Read the model definition and answer for the solid it produces. Units are mm, in the model's axes. Coordinates: 2 decimals unless noted, no trailing zeros. Order: outer loops, then holes, each group sorted by start corner. A loop starts at its lowest first (then second) coordinate and runs counter-clockwise, first axis right, second up.
Autodesk Inventor part; units mm, degrees
ref_plane "YZ Plane" through (0, 0, 0) normal (1, 0, 0) x (0, 1, 0)
ref_plane "XZ Plane" through (0, 0, 0) normal (0, 1, 0) x (-1, 0, 0)
ref_plane "XY Plane" through (0, 0, 0) normal (0, 0, 1) x (1, 0, 0)
sketch "Sketch1" plane through (0, 0, 0) normal (0, 1, 0) x (-1, 0, 0)
  line L0 (7.366, 6.1452) -> (7.366, -23.8548)
  line L1 (7.366, -23.8548) -> (0, -23.8548)
  line L2 (6.096, -8.0476) -> (6.096, -9.0212)
  line L3 (0, 0.4868) -> (0, 3.5348)
  line L4 (6.096, 3.5348) -> (6.096, -8.0476)
  line L5 (0, -9.0212) -> (0, -11.8152)
  line L6 (6.096, -12.0692) -> (6.096, -9.0212)
  line L7 (6.096, 3.5348) -> (0, 0.4868)
  line L8 (6.096, -12.0692) -> (0, -9.0212)
  line L9 (0, -23.8548) -> (0, -9.0212)
  line L10 (0, 0.4868) -> (0, 16.3788)
  line L11 (6.096, 13.3308) -> (6.096, 16.3788)
  line L12 (6.096, 13.3308) -> (0, 16.3788)
  line L13 (6.096, 28.9348) -> (6.096, 17.3524)
  line L14 (6.096, 28.9348) -> (0, 25.8868)
  line L15 (6.096, 17.3524) -> (6.096, 16.3788)
  line L16 (6.096, 38.7308) -> (6.096, 41.7788)
  line L17 (6.096, 38.7308) -> (0, 41.7788)
  line L18 (6.096, 54.3348) -> (6.096, 42.7524)
  line L19 (6.096, 54.3348) -> (0, 51.2868)
  line L20 (6.096, 42.7524) -> (6.096, 41.7788)
  line L21 (6.096, 64.1308) -> (6.096, 67.1788)
  line L22 (6.096, 64.1308) -> (0, 67.1788)
  line L23 (6.096, 79.7348) -> (6.096, 68.1524)
  line L24 (6.096, 79.7348) -> (0, 76.6868)
  line L25 (6.096, 68.1524) -> (6.096, 67.1788)
  line L26 (7.366, 6.1452) -> (7.366, 91.622)
  line L27 (7.366, 91.622) -> (0, 91.622)
  line L28 (0, 25.8868) -> (0, 41.7788)
  line L29 (0, 51.2868) -> (0, 67.1788)
  line L30 (0, 76.6868) -> (0, 91.622)
  line L31 (6.096, -4.2672) -> (4.0009, -4.2672) construction
  point P0 (0, 0)
  dimension "d0" = 7.366
  dimension "d8" = 9.508
  dimension "d10" = 3.048
  dimension "d11" = 3.048
  dimension "d12" = 6.096
  dimension "d17" = 25.4
  dimension "d24" = 11.7856
  dimension "d67" = 115.4768
  dimension "d70" = 23.8548
  dimension "d71" = 4.754
extrude "MultipleTeeth" add sketch "Sketch1" along normal blind 19.05
sketch "Sketch2" plane through (0, 0, 0) normal (0, -1, 0) x (1, 0, 0)
  line L0 (0, 0.4868) -> (-6.096, 3.5348) construction
  line L1 (-6.096, 3.5348) -> (-6.096, -12.0692) construction
  line L2 (-6.096, -12.0692) -> (0, -9.0212) construction
  line L3 (0, 16.3788) -> (0, 0.4868)
  line L4 (0, 0.4868) -> (-6.096, 3.5348)
  line L5 (-6.096, -12.0692) -> (0, -9.0212)
  line L6 (-6.096, 3.5348) -> (-6.096, -12.0692)
  line L7 (-6.096, -12.0692) -> (-6.096, 3.5348)
  line L8 (0, -9.0212) -> (-6.096, -12.0692)
  line L9 (-7.366, -23.8548) -> (-7.366, 91.622)
  line L10 (-7.366, -59.508) -> (-7.366, -32.8548)
  line L11 (-7.366, -23.8548) -> (0, -23.8548)
  line L12 (-7.366, 91.622) -> (0, 91.622)
  line L13 (-7.366, -55.8503) -> (-7.366, -40.458) construction
  line L14 (0, -43.0234) -> (0, -59.508) construction
  line L15 (-6.096, -62.0648) -> (0, -62.0648) construction
  line L16 (0, -32.8548) -> (0, -37.6258)
  line L17 (0, -49.9828) -> (0, -62.0648)
  line L18 (0, -62.0648) -> (0, -59.508)
  line L19 (0, -32.8548) -> (-7.366, -32.8548) construction
  line L20 (0, -51.9048) -> (-7.366, -51.9048) construction
  line L21 (0, -42.3798) -> (-7.366, -42.3798) construction
  line L22 (-6.096, -12.0692) -> (-6.096, -62.0648) construction
  line L23 (0, -37.6258) -> (-6.096, -34.5778)
  line L24 (-6.096, -50.1818) -> (-6.096, -34.5778)
  line L25 (0, -47.1338) -> (-6.096, -50.1818)
  line L26 (0, -9.0212) -> (0, -23.8548)
  line L27 (0, -23.8548) -> (0, -32.8548)
  line L28 (-7.366, -32.8548) -> (-7.366, -23.8548)
  line L29 (0, -49.9828) -> (0, -47.1338)
  line L30 (0, -62.0648) -> (-7.366, -62.0648)
  line L31 (-7.366, -62.0648) -> (-7.366, -59.508)
  point P0 (0, 0)
  dimension "d25" = 115.4768
  dimension "d33" = 9
  dimension "d34" = 19.05
  dimension "d36" = 9.525
  dimension "d38" = 10.16
extrude "LongTooth" add sketch "Sketch2" against normal blind 100.2792
sketch "Sketch3" plane through (0, 19.05, 0) normal (0, 1, 0) x (1, 0, 0)
  line L0 (-6.096, -3.5348) -> (-6.096, 12.0692) construction
  line L1 (0, 23.8548) -> (-7.366, 23.8548)
  line L2 (-7.366, -91.622) -> (0, -91.622)
  line L3 (-7.366, 23.8548) -> (-6.096, 23.8548)
  line L4 (-6.096, 23.8548) -> (-6.096, -91.622)
  line L5 (-6.096, -91.622) -> (-7.366, -91.622)
  line L6 (-7.366, -91.622) -> (-7.366, 23.8548)
  point P0 (0, 0)
extrude "ThinPlate" add sketch "Sketch3" along normal up to surface (81.2292 mm away)
sketch "Sketch4" plane through (0, 0, 0) normal (0, -1, 0) x (1, 0, 0)
  line L0 (-6.096, 91.622) -> (0, 91.622)
  line L1 (-7.366, 91.622) -> (-7.366, -62.0648)
  line L2 (0, 91.622) -> (-7.366, 91.622)
  line L3 (-7.366, 91.622) -> (-7.366, -62.0648)
  line L4 (-7.366, -62.0648) -> (0, -62.0648)
  line L5 (0, -62.0648) -> (0, 91.622)
  point P0 (0, 0)
extrude "Extrusion4" add sketch "Sketch4" along normal blind 5.08
ref_plane "Work Plane1" through (-15.892, 0, 8.4328) normal (0, 0, 1) x (0, 1, 0)
sketch "Sketch6" plane through (0, 19.05, 16.3788) normal (1, 0, 0) x (0, 0, -1)
  circle A0 centre (71.4586, -8.89) radius 1.9304
  line L0 (78.4436, 81.2292) -> (78.4436, -24.13)
  line L1 (78.4436, -24.13) -> (-75.2432, -24.13)
  circle A1 centre (58.7586, -8.89) radius 1.9304
  circle A2 centre (46.0586, -8.89) radius 1.9304
  circle A3 centre (71.4586, 3.81) radius 1.9304
  circle A4 centre (58.7586, 3.81) radius 1.9304
  circle A5 centre (46.0586, 3.81) radius 1.9304
  circle A6 centre (71.4586, 16.51) radius 1.9304
  circle A7 centre (58.7586, 16.51) radius 1.9304
  circle A8 centre (46.0586, 16.51) radius 1.9304
  circle A9 centre (71.4586, 29.21) radius 1.9304
  circle A10 centre (58.7586, 29.21) radius 1.9304
  circle A11 centre (46.0586, 29.21) radius 1.9304
  circle A12 centre (71.4586, 41.91) radius 1.9304
  circle A13 centre (58.7586, 41.91) radius 1.9304
  circle A14 centre (46.0586, 41.91) radius 1.9304
  circle A15 centre (71.4586, 54.61) radius 1.9304
  circle A16 centre (58.7586, 54.61) radius 1.9304
  circle A17 centre (46.0586, 54.61) radius 1.9304
  circle A18 centre (71.4586, 67.31) radius 1.9304
  circle A19 centre (58.7586, 67.31) radius 1.9304
  circle A20 centre (46.0586, 67.31) radius 1.9304
  circle A21 centre (71.4586, 80.01) radius 1.9304
  circle A22 centre (58.7586, 80.01) radius 1.9304
  circle A23 centre (46.0586, 80.01) radius 1.9304
  circle A24 centre (33.3586, -8.89) radius 1.9304
  circle A25 centre (33.3586, 3.81) radius 1.9304
  circle A26 centre (33.3586, 16.51) radius 1.9304
  circle A27 centre (33.3586, 29.21) radius 1.9304
  circle A28 centre (33.3586, 41.91) radius 1.9304
  circle A29 centre (33.3586, 54.61) radius 1.9304
  circle A30 centre (33.3586, 67.31) radius 1.9304
  circle A31 centre (33.3586, 80.01) radius 1.9304
  circle A32 centre (20.6586, -8.89) radius 1.9304
  circle A33 centre (20.6586, 3.81) radius 1.9304
  circle A34 centre (20.6586, 16.51) radius 1.9304
  circle A35 centre (20.6586, 29.21) radius 1.9304
  circle A36 centre (20.6586, 41.91) radius 1.9304
  circle A37 centre (20.6586, 54.61) radius 1.9304
  circle A38 centre (20.6586, 67.31) radius 1.9304
  circle A39 centre (20.6586, 80.01) radius 1.9304
  circle A40 centre (7.9586, -8.89) radius 1.9304
  circle A41 centre (7.9586, 3.81) radius 1.9304
  circle A42 centre (7.9586, 16.51) radius 1.9304
  circle A43 centre (7.9586, 29.21) radius 1.9304
  circle A44 centre (7.9586, 41.91) radius 1.9304
  circle A45 centre (7.9586, 54.61) radius 1.9304
  circle A46 centre (7.9586, 67.31) radius 1.9304
  circle A47 centre (7.9586, 80.01) radius 1.9304
  circle A48 centre (-4.7414, -8.89) radius 1.9304
  circle A49 centre (-4.7414, 3.81) radius 1.9304
  circle A50 centre (-4.7414, 16.51) radius 1.9304
  circle A51 centre (-4.7414, 29.21) radius 1.9304
  circle A52 centre (-4.7414, 41.91) radius 1.9304
  circle A53 centre (-4.7414, 54.61) radius 1.9304
  circle A54 centre (-4.7414, 67.31) radius 1.9304
  circle A55 centre (-4.7414, 80.01) radius 1.9304
  circle A56 centre (-17.4414, -8.89) radius 1.9304
  circle A57 centre (-17.4414, 3.81) radius 1.9304
  circle A58 centre (-17.4414, 16.51) radius 1.9304
  circle A59 centre (-17.4414, 29.21) radius 1.9304
  circle A60 centre (-17.4414, 41.91) radius 1.9304
  circle A61 centre (-17.4414, 54.61) radius 1.9304
  circle A62 centre (-17.4414, 67.31) radius 1.9304
  circle A63 centre (-17.4414, 80.01) radius 1.9304
  circle A64 centre (-30.1414, -8.89) radius 1.9304
  circle A65 centre (-30.1414, 3.81) radius 1.9304
  circle A66 centre (-30.1414, 16.51) radius 1.9304
  circle A67 centre (-30.1414, 29.21) radius 1.9304
  circle A68 centre (-30.1414, 41.91) radius 1.9304
  circle A69 centre (-30.1414, 54.61) radius 1.9304
  circle A70 centre (-30.1414, 67.31) radius 1.9304
  circle A71 centre (-30.1414, 80.01) radius 1.9304
  circle A72 centre (-42.8414, -8.89) radius 1.9304
  circle A73 centre (-42.8414, 3.81) radius 1.9304
  circle A74 centre (-42.8414, 16.51) radius 1.9304
  circle A75 centre (-42.8414, 29.21) radius 1.9304
  circle A76 centre (-42.8414, 41.91) radius 1.9304
  circle A77 centre (-42.8414, 54.61) radius 1.9304
  circle A78 centre (-42.8414, 67.31) radius 1.9304
  circle A79 centre (-42.8414, 80.01) radius 1.9304
  circle A80 centre (-55.5414, -8.89) radius 1.9304
  circle A81 centre (-55.5414, 3.81) radius 1.9304
  circle A82 centre (-55.5414, 16.51) radius 1.9304
  circle A83 centre (-55.5414, 29.21) radius 1.9304
  circle A84 centre (-55.5414, 41.91) radius 1.9304
  circle A85 centre (-55.5414, 54.61) radius 1.9304
  circle A86 centre (-55.5414, 67.31) radius 1.9304
  circle A87 centre (-55.5414, 80.01) radius 1.9304
  circle A88 centre (-68.2414, -8.89) radius 1.9304
  circle A89 centre (-68.2414, 3.81) radius 1.9304
  circle A90 centre (-68.2414, 16.51) radius 1.9304
  circle A91 centre (-68.2414, 29.21) radius 1.9304
  circle A92 centre (-68.2414, 41.91) radius 1.9304
  circle A93 centre (-68.2414, 54.61) radius 1.9304
  circle A94 centre (-68.2414, 67.31) radius 1.9304
  circle A95 centre (-68.2414, 80.01) radius 1.9304
  circle A96 centre (-80.9414, -8.89) radius 1.9304
  circle A97 centre (-80.9414, 3.81) radius 1.9304
  circle A98 centre (-80.9414, 16.51) radius 1.9304
  circle A99 centre (-80.9414, 29.21) radius 1.9304
  circle A100 centre (-80.9414, 41.91) radius 1.9304
  circle A101 centre (-80.9414, 54.61) radius 1.9304
  circle A102 centre (-80.9414, 67.31) radius 1.9304
  circle A103 centre (-80.9414, 80.01) radius 1.9304
  point P0 (16.3788, -19.05)
  dimension "d56" = 3.8608
  dimension "d57" = 6.985
  dimension "d58" = 15.24
  dimension "d61" = 12.7
  dimension "d64" = 12.7
equation "\"d11\" = d10"
equation "\"d71\" = 0.5 * d8"
equation "\"d36\" = 0.5 * d34"
properties part number "Lift receiver left side actobtics"
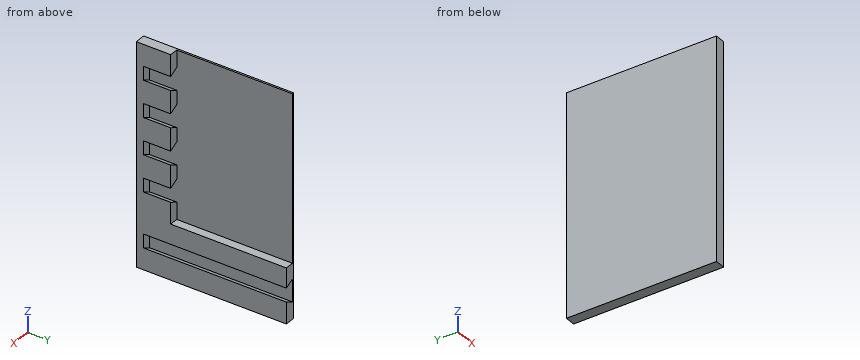
1) A cutting plane is placed at D-D, the plane y = 67. Determine the outline of the cut face in (x, z).
A:
outline: (-7.37, -62.06) - (0, -62.06) - (0, -47.13) - (-6.1, -50.18) - (-6.1, -34.58) - (0, -37.63) - (0, -23.85) - (-6.1, -23.85) - (-6.1, 91.62) - (-7.37, 91.62) - close
2) A cutting plane is placed at A-A, the plane y = 10.5. Determine the outline of the cut face in (x, z).
A:
outline: (-7.37, -62.06) - (0, -62.06) - (0, -47.13) - (-6.1, -50.18) - (-6.1, -34.58) - (0, -37.63) - (0, -9.02) - (-6.1, -12.07) - (-6.1, 3.53) - (0, 0.49) - (0, 16.38) - (-6.1, 13.33) - (-6.1, 28.93) - (0, 25.89) - (0, 41.78) - (-6.1, 38.73) - (-6.1, 54.33) - (0, 51.29) - (0, 67.18) - (-6.1, 64.13) - (-6.1, 79.73) - (0, 76.69) - (0, 91.62) - (-7.37, 91.62) - close
3) Flat-ended cylindrical pins translate along their axes: pin 1 Ø1.8 at (x, z) = (-2, 85.5) entering from +Y; pin 2 Ø1.8 at (x, z) = (-3.5, 70) entering from +Y; pin 3 Ø8 at (y, z) = (65, -42) entering from +X. Find the tip coordinate at first contact, or state that the pin passes through.
A:
pin 1: stops at y = 19.05
pin 2: stops at y = 0
pin 3: stops at x = -6.1
4) Straight lines are drawn through the part: line 1 (X direction, y = 34, z = 81); line 2 (Y direction, x = -1.5, z = 27); line 3 (Y direction, x = -4, z = 71.5). For each, find the intervals that lie inside material, in ascending order.
A:
line 1: x = -7.37 to -6.1
line 2: y = -5.08 to 19.05
line 3: y = -5.08 to 0
5) A cutting plane is placed at B-B, the plane x = -2.75. Determine the outline of the cut face in (y, z).
A:
outline: (-5.08, -62.06) - (100.28, -62.06) - (100.28, -48.51) - (0, -48.51) - (0, -36.25) - (100.28, -36.25) - (100.28, -23.85) - (19.05, -23.85) - (19.05, -10.4) - (0, -10.4) - (0, 1.86) - (19.05, 1.86) - (19.05, 15) - (0, 15) - (0, 27.26) - (19.05, 27.26) - (19.05, 40.4) - (0, 40.4) - (0, 52.66) - (19.05, 52.66) - (19.05, 65.8) - (0, 65.8) - (0, 78.06) - (19.05, 78.06) - (19.05, 91.62) - (-5.08, 91.62) - close
6) A cutting plane is placed at C-C, the plane z = -2. Determine the outline of the cut face in (x, y), and give its area (3 significant figures).
A:
outline: (-7.37, -5.08) - (0, -5.08) - (0, 0) - (-6.1, 0) - (-6.1, 100.28) - (-7.37, 100.28) - close
area: 165 mm2
